Work out the finished part from the listing and answer in its coordinate system (mm). Face numbers are marked on the shaded views. A direction names the side the tool comes from. Coordinates: 2 decimals unless noted, no trailing zeros. Write each loop counter-clockwise with the first axis right and the second up, starting at its lowest first coordinate (ties: lowest second). Pieces come first, ordered by that corner, then holes. Notation, with made-up numbers: (-30.5, 72) - (21.5, 72) arc R23 cw to (21.5, 102) - close; hole circle Ø6 at (-14.75, -11). An arc over 180 degrees is marked (long way). One line per item, written item: value.
```python
from build123d import *

# Parameters (mm, degrees)
SKETCH_1_R                    = 1.25
EXTRUDE_1_DEPTH               = 4
HOLE_WIZARD_M2_5_1_AT_2_COUNT = 2
HOLE_WIZARD_M2_5_1_AT_2_PITCH = 18
HOLE_WIZARD_M2_5_1_AT_3_COUNT = 2
HOLE_WIZARD_M2_5_1_AT_3_PITCH = 36
SKETCH_7_W                    = 66
SKETCH_7_H                    = 10
EXTRUDE_2_DEPTH               = 4
SKETCH_7_3_R                  = 2.5
CUT_EXTRUDE_1_DEPTH           = 4
HOLE_WIZARD_M2_5_2_D          = 2.05
HOLE_WIZARD_M2_5_2_DEPTH      = 7.25
HOLE_WIZARD_M2_5_2_TIP        = 0.615882135


with BuildPart() as part:
    # 草图1 → 凸台-拉伸1 (new body)
    with BuildSketch(Plane(origin=(0, 0, 0), x_dir=(1, 0, 0), z_dir=(0, 1, 0))):
        Polygon((0, 0), (0, 43), (66, 43), (66, -43), (0, -43), align=None)
        with Locations((2, 0)):
            Circle(SKETCH_1_R, mode=Mode.SUBTRACT)
        with Locations((2, 35)):
            Circle(SKETCH_1_R, mode=Mode.SUBTRACT)
        with Locations((2, -35)):
            Circle(SKETCH_1_R, mode=Mode.SUBTRACT)
    extrude(amount=EXTRUDE_1_DEPTH)

    # 草图6 → M2.5 螺纹孔1 (revolve, cut)
    with BuildSketch(Plane(origin=(15, 2, 43), x_dir=(0, -1, 0), z_dir=(1, 0, 0))):
        Polygon((0, 0), (0, 8.865882135), (1.025, 8.25), (1.025, 0), align=None)
    hole_wizard_m2_5_1 = revolve(axis=Axis((15, 2, 49.35), (0, 0, -1)), mode=Mode.SUBTRACT)

    # M2.5 螺纹孔1 at 2: M2.5 螺纹孔1 ×2
    with Locations(*[(i * HOLE_WIZARD_M2_5_1_AT_2_PITCH, 0, 0) for i in range(1, HOLE_WIZARD_M2_5_1_AT_2_COUNT)]):
        add(hole_wizard_m2_5_1, mode=Mode.SUBTRACT)

    # M2.5 螺纹孔1 at 3: M2.5 螺纹孔1 ×2
    with Locations(*[(i * HOLE_WIZARD_M2_5_1_AT_3_PITCH, 0, 0) for i in range(1, HOLE_WIZARD_M2_5_1_AT_3_COUNT)]):
        add(hole_wizard_m2_5_1, mode=Mode.SUBTRACT)

    # 镜向1: M2.5 螺纹孔1 across plane
    add(hole_wizard_m2_5_1.mirror(Plane.XY), mode=Mode.SUBTRACT)

    # 镜向1 copy 1 sketch → 镜向1 copy 1 (revolve, cut)
    with BuildSketch(Plane(origin=(33, 2, -43), x_dir=(0, -1, 0), z_dir=(1, 0, 0))):
        Polygon((0, 0), (0, -8.865882135), (1.025, -8.25), (1.025, 0), align=None)
    revolve(axis=Axis((33, 2, -49.35), (0, 0, -1)), mode=Mode.SUBTRACT)

    # 镜向1 copy 2 sketch → 镜向1 copy 2 (revolve, cut)
    with BuildSketch(Plane(origin=(51, 2, -43), x_dir=(0, -1, 0), z_dir=(1, 0, 0))):
        Polygon((0, 0), (0, -8.865882135), (1.025, -8.25), (1.025, 0), align=None)
    revolve(axis=Axis((51, 2, -49.35), (0, 0, -1)), mode=Mode.SUBTRACT)

    # 草图7 → 凸台-拉伸2 (add)
    with BuildSketch(Plane(origin=(0, 4, 0), x_dir=(1, 0, 0), z_dir=(0, 1, 0))):
        with Locations((33, 21.5)):
            Rectangle(SKETCH_7_W, SKETCH_7_H)
        with Locations((33, -21.5)):
            Rectangle(SKETCH_7_W, SKETCH_7_H)
    extrude(amount=EXTRUDE_2_DEPTH)

    # 草图7<3> → 切除-拉伸1 (cut, symmetric)
    with BuildSketch(Plane(origin=(0, 4, 0), x_dir=(1, 0, 0), z_dir=(0, 1, 0))):
        with Locations((13, 21.5)):
            Circle(SKETCH_7_3_R)
        with Locations((53, 21.5)):
            Circle(SKETCH_7_3_R)
        with Locations((53, -21.5)):
            Circle(SKETCH_7_3_R)
        with Locations((13, -21.5)):
            Circle(SKETCH_7_3_R)
    extrude(amount=CUT_EXTRUDE_1_DEPTH, both=True, mode=Mode.SUBTRACT)

    # M2.5 螺纹孔2
    with Locations(Plane(origin=(66, 0, 0), x_dir=(0, 0, -1), z_dir=(1, 0, 0))):
        with Locations((-35, 2), (0, 2), (35, 2)):
            Hole(HOLE_WIZARD_M2_5_2_D / 2, depth=HOLE_WIZARD_M2_5_2_DEPTH)
            with Locations((0, 0, -(HOLE_WIZARD_M2_5_2_DEPTH + HOLE_WIZARD_M2_5_2_TIP / 2))):  # 118° drill point
                Cone(0, HOLE_WIZARD_M2_5_2_D / 2, HOLE_WIZARD_M2_5_2_TIP, mode=Mode.SUBTRACT)


solid = part.part
```
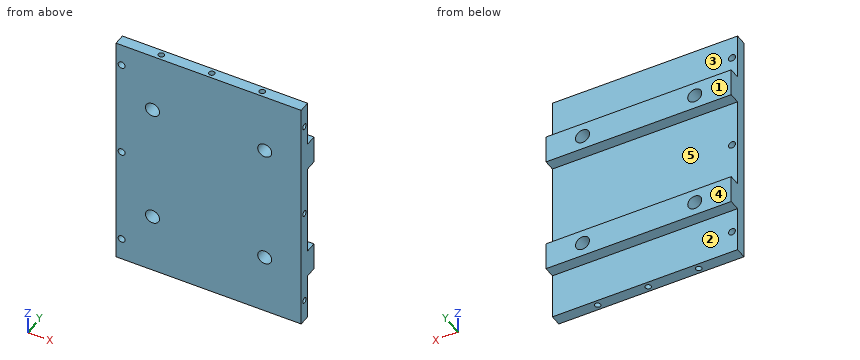
Item 1: Section D-D, the plane z = -22.5 is taken. Determine the outline of the cut face in (x, y), then the cut area to 3 significant figures.
Evaluation:
outline: (0, 0) - (10.71, 0) - (10.71, 8) - (0, 8) - close; (15.29, 0) - (50.71, 0) - (50.71, 8) - (15.29, 8) - close; (55.29, 0) - (66, 0) - (66, 8) - (55.29, 8) - close
area: 455 mm2
Item 2: Section A-A, the plane y = 5.5 is taken. Determine the outline of the cut face in (x, z), then the cut area to 3 significant figures.
Evaluation:
outline: (0, -26.5) - (66, -26.5) - (66, -16.5) - (0, -16.5) - close; (0, 16.5) - (66, 16.5) - (66, 26.5) - (0, 26.5) - close; hole circle Ø5 at (13, -21.5); hole circle Ø5 at (13, 21.5); hole circle Ø5 at (53, -21.5); hole circle Ø5 at (53, 21.5)
area: 1,240 mm2
Item 3: Which of the six approach directions +Z, -Z, +X, -X, +Y, -Y give full straight-line access (tool end or side, diameter ignored) to the marked faces 1, 2 and 3?
Evaluation:
face 1: +Z, -Z, +X, -X, +Y
face 2: -Z, +X, -X, +Y
face 3: +Z, +X, -X, +Y
Item 4: Determine the mould class of the marked faces 4 and 5 for opening direction Z: +Z half, -Z half, draft (parallel to the pull), parting line (faces both ways), or undercut.
Evaluation:
face 4: draft
face 5: undercut
Item 5: Given pin 1 (1 mm diameter, centred on x = 42.5, y = 7, fed in from -Z); pin 2 (3 mm diameter, centred on x = 2, z = 0, fed in from +Y); pin 3 (1.2 mm diameter, centred on x = 35, y = 5, fed in from +Z), each flat-ended and moving along its own axis, determine where each tip first touches the part or whether it passes through.
Evaluation:
pin 1: stops at z = -26.5
pin 2: stops at y = 4
pin 3: stops at z = 26.5
Item 6: Section C-C, the plane x = 53 is taken. Determine the outline of the cut face in (y, z), then the cut area to 3 significant figures.
Evaluation:
outline: (0, -43) - (4, -43) - (4, -26.5) - (8, -26.5) - (8, -24) - (0, -24) - close; (0, -19) - (8, -19) - (8, -16.5) - (4, -16.5) - (4, 16.5) - (8, 16.5) - (8, 19) - (0, 19) - close; (0, 24) - (8, 24) - (8, 26.5) - (4, 26.5) - (4, 43) - (0, 43) - close
area: 344 mm2
Item 7: Consider probe 1 along X at (y, z) = (2, -39.5) (3 decimals); probe 2 along X at (y, z) = (4.75, -21.5); probe 3 along Z at (x, y) = (13, 6.25). Determine where each line is inside the solid, lowest interval first.
Evaluation:
probe 1: x = 0 to 13.975, 16.025 to 31.975, 34.025 to 49.975, 52.025 to 66
probe 2: x = 0 to 10.5, 15.5 to 50.5, 55.5 to 66
probe 3: z = -26.5 to -24, -19 to -16.5, 16.5 to 19, 24 to 26.5
Item 8: Section B-B, the plane x = 2 is taken. Determine the outline of the cut face in (y, z), then the cut area to 3 significant figures.
Evaluation:
outline: (0, -43) - (4, -43) - (4, -36.25) - (0, -36.25) - close; (0, -33.75) - (4, -33.75) - (4, -26.5) - (8, -26.5) - (8, -16.5) - (4, -16.5) - (4, -1.25) - (0, -1.25) - close; (0, 1.25) - (4, 1.25) - (4, 16.5) - (8, 16.5) - (8, 26.5) - (4, 26.5) - (4, 33.75) - (0, 33.75) - close; (0, 36.25) - (4, 36.25) - (4, 43) - (0, 43) - close
area: 394 mm2
